from build123d import *

# Parameters (mm, degrees)
SCHIZZO1_R                   = 2.1
ESTRUSIONE_ESTRUSIONE1_DEPTH = 500
SCHIZZO2_R                   = 3
TAGLIO_ESTRUSIONE1_DEPTH     = 15


with BuildPart() as part:
    # Schizzo1 → Estrusione-Estrusione1 (new body)
    with BuildSketch(Plane.XY):
        with BuildLine():
            Line((-3.6, 0), (-4, 0.4))
            Line((-4, 0.4), (-4, 3))
            Line((-4, 3), (-7, 6))
            Line((-7, 6), (-8, 6))
            Line((-8, 6), (-8, 3))
            Line((-8, 3), (-9.5, 3))
            ThreePointArc((-9.5, 3), (-9.853553391, 3.146446609), (-10, 3.5))
            Line((-10, 3.5), (-10, 9))
            ThreePointArc((-10, 9), (-9.707106781, 9.707106781), (-9, 10))
            Line((-9, 10), (-3.5, 10))
            ThreePointArc((-3.5, 10), (-3.146446609, 9.853553391), (-3, 9.5))
            Line((-3, 9.5), (-3, 8))
            Line((-3, 8), (-6, 8))
            Line((-6, 8), (-6, 7))
            Line((-6, 7), (-3, 4))
            Line((-3, 4), (-0.4, 4))
            Line((-0.4, 4), (0, 3.6))
            Line((0, 3.6), (0.4, 4))
            Line((0.4, 4), (3, 4))
            Line((3, 4), (6, 7))
            Line((6, 7), (6, 8))
            Line((6, 8), (3, 8))
            Line((3, 8), (3, 9.5))
            ThreePointArc((3, 9.5), (3.146446609, 9.853553391), (3.5, 10))
            Line((3.5, 10), (9, 10))
            ThreePointArc((9, 10), (9.707106781, 9.707106781), (10, 9))
            Line((10, 9), (10, 3.5))
            ThreePointArc((10, 3.5), (9.853553391, 3.146446609), (9.5, 3))
            Line((9.5, 3), (8, 3))
            Line((8, 3), (8, 6))
            Line((8, 6), (7, 6))
            Line((7, 6), (4, 3))
            Line((4, 3), (4, 0.4))
            Line((4, 0.4), (3.6, 0))
            Line((3.6, 0), (4, -0.4))
            Line((4, -0.4), (4, -3))
            Line((4, -3), (7, -6))
            Line((7, -6), (8, -6))
            Line((8, -6), (8, -3))
            Line((8, -3), (9.5, -3))
            ThreePointArc((9.5, -3), (9.853553391, -3.146446609), (10, -3.5))
            Line((10, -3.5), (10, -9))
            ThreePointArc((10, -9), (9.707106781, -9.707106781), (9, -10))
            Line((9, -10), (3.5, -10))
            ThreePointArc((3.5, -10), (3.146446609, -9.853553391), (3, -9.5))
            Line((3, -9.5), (3, -8))
            Line((3, -8), (6, -8))
            Line((6, -8), (6, -7))
            Line((6, -7), (3, -4))
            Line((3, -4), (0.4, -4))
            Line((0.4, -4), (0, -3.6))
            Line((0, -3.6), (-0.4, -4))
            Line((-0.4, -4), (-3, -4))
            Line((-3, -4), (-6, -7))
            Line((-6, -7), (-6, -8))
            Line((-6, -8), (-3, -8))
            Line((-3, -8), (-3, -9.5))
            ThreePointArc((-3, -9.5), (-3.146446609, -9.853553391), (-3.5, -10))
            Line((-3.5, -10), (-9, -10))
            ThreePointArc((-9, -10), (-9.707106781, -9.707106781), (-10, -9))
            Line((-10, -9), (-10, -3.5))
            ThreePointArc((-10, -3.5), (-9.853553391, -3.146446609), (-9.5, -3))
            Line((-9.5, -3), (-8, -3))
            Line((-8, -3), (-8, -6))
            Line((-8, -6), (-7, -6))
            Line((-7, -6), (-4, -3))
            Line((-4, -3), (-4, -0.4))
            Line((-4, -0.4), (-3.6, 0))
        make_face()
        Circle(SCHIZZO1_R, mode=Mode.SUBTRACT)
    extrude(amount=ESTRUSIONE_ESTRUSIONE1_DEPTH)

    # Schizzo2 → Taglio-Estrusione1 (cut, through all)
    with BuildSketch(Plane.ZY.offset(4)):
        with Locations((25, 0)):
            Circle(SCHIZZO2_R)
        with Locations((475, 0)):
            Circle(SCHIZZO2_R)
    extrude(amount=-TAGLIO_ESTRUSIONE1_DEPTH, mode=Mode.SUBTRACT)


solid = part.part
CAD build for the part. Positions are in the model's coordinates, mm. Round coordinates to 2 decimals unless told otherwise and drop trailing zeros. Write item = value, one per line. Start each with the question number.
(1) Pin check, flat tips, straight feed: P1, Ø0.8, axis at y = 2, z = 314, coming from the +X side; P2, Ø0.8, axis at x = -2, z = 151, coming from the -Y side. Stop position of each tip, or through.
(2) Pull direction Z, two halves, no side cores. Call faces 1 (the flat face through (0.1, 2.4, 500)), 2 (the flat face through (0.1, 2.4, 0)): released by +Z, released by -Z, zero draft, split by the parting line, or undercut.
(3) Probe line 1 (Y direction, x = -5, z = 178); line 2 (Z direction, x = -3.75, y = 0.25); line 3 (X direction, y = -8.5, z = 86). List the from-to ranges inside material, lowest first. Write a range as [from, to].
Model answer:
q1.P1 = 4
q1.P2 = -4
q2.face_1 = released by +Z
q2.face_2 = released by -Z
q3.line_1 = [-10, -8], [-6, -4], [4, 6], [8, 10]
q3.line_2 = [0, 22.01], [27.99, 472.01], [477.99, 500]
q3.line_3 = [-10, -3], [3, 10]
